Autodesk Inventor part; units mm, degrees
ref_plane "Work Plane1" through (55.8263, 1.3, -122.3626) normal (1, 0, 0) x (0, 0, -1)
ref_plane "Work Plane2" through (56.5713, 0, -122.3626) normal (-1, 0, 0) x (0, 0, 1)
ref_plane "Work Plane3" through (0, 0.5, 0) normal (0, -1, 0) x (1, 0, 0)
sketch "Sketch1" plane through (0, 0, 0) normal (0, 1, 0) x (-1, 0, 0)
  line L0 (-52.5263, -125.0626) -> (-59.1263, -125.0626)
  line L1 (-59.1263, -125.0626) -> (-59.1263, -122.3626)
  line L2 (-59.1263, -122.3626) -> (-52.5263, -122.3626)
  line L3 (-52.5263, -122.3626) -> (-52.5263, -125.0626)
  dimension "d0" = 6.6
  dimension "d1" = 2.7
extrude "Extrusion1" add sketch "Sketch1" along normal blind 1.3
sketch "Sketch2" plane through (52.5263, 0, -122.3626) normal (0, 0, 1) x (1, 0, 0)
  line L0 (6.6, 0) -> (6.6, 1.3)
  line L1 (6.6, 1.3) -> (4.67, 1.3)
  line L2 (0, 1.3) -> (6.6, 1.3)
  line L3 (0, 0) -> (6.6, 0)
  line L4 (4.67, 0) -> (3.42, 0)
  line L5 (3.42, 0) -> (3.42, 1)
  line L6 (3.42, 1) -> (4.67, 1)
  line L7 (4.67, 1) -> (4.67, 0)
  point P0 (3.42, 0)
  dimension "d4" = 1.93
  dimension "d5" = 1.25
  dimension "d6" = 1
extrude "Extrusion2" add sketch "Sketch2" along normal blind 1.5
sketch "Sketch3" plane through (0, 0, 0) normal (0, -1, 0) x (1, 0, 0)
  line L0 (55.8263, -125.0626) -> (55.8263, -126.2505)
  line L1 (52.5263, -125.0626) -> (52.0463, -125.0626)
  line L2 (52.0463, -125.0626) -> (52.0463, -124.6026)
  line L3 (52.0463, -124.6026) -> (52.5263, -124.6026)
  line L4 (52.5263, -122.3626) -> (52.0463, -122.3626)
  line L5 (52.0463, -122.3626) -> (52.0463, -122.8226)
  line L6 (52.0463, -122.8226) -> (52.5263, -122.8226)
  line L7 (59.1263, -125.0626) -> (59.6063, -125.0626)
  line L8 (59.6063, -125.0626) -> (59.6063, -124.6026)
  line L9 (59.6063, -124.6026) -> (59.1263, -124.6026)
  line L10 (59.1263, -122.3626) -> (59.6063, -122.3626)
  line L11 (59.6063, -122.3626) -> (59.6063, -122.8226)
  line L12 (59.6063, -122.8226) -> (59.1263, -122.8226)
  line L13 (52.5263, -126.3425) -> (53.2263, -126.3425)
  line L14 (59.1263, -125.0626) -> (59.1263, -125.9026)
  line L15 (59.1263, -122.3626) -> (59.1263, -122.8226)
  line L16 (59.1263, -124.6026) -> (59.1263, -125.0626)
  line L17 (52.5263, -125.0626) -> (52.5263, -124.6026)
  line L18 (52.5263, -122.8226) -> (52.5263, -122.3626)
  line L19 (59.1263, -125.0626) -> (52.5263, -125.0626)
  line L20 (53.2263, -125.9026) -> (53.6263, -125.9026)
  line L21 (53.6263, -125.9026) -> (53.6263, -125.0626)
  line L22 (53.6263, -125.0626) -> (53.2263, -125.0626)
  line L23 (53.2263, -125.0626) -> (53.2263, -125.9026)
  line L24 (58.4263, -125.9026) -> (58.0263, -125.9026)
  line L25 (58.0263, -125.9026) -> (58.0263, -125.0626)
  line L26 (58.0263, -125.0626) -> (58.4263, -125.0626)
  line L27 (58.4263, -125.0626) -> (58.4263, -125.9026)
  line L28 (58.0263, -125.9026) -> (57.0263, -125.9026)
  line L29 (56.6263, -125.0626) -> (57.0263, -125.0626)
  line L30 (57.0263, -125.0626) -> (57.0263, -125.9026)
  line L31 (56.6263, -125.9026) -> (56.6263, -125.0626)
  line L32 (57.0263, -125.9026) -> (56.6263, -125.9026)
  dimension "d15" = 0.4
  dimension "d16" = 1
extrude "Extrusion3" add sketch "Sketch3" against normal blind 0.2 contours L1 L2 L3 L17 | L16 L9 L8 L7 | L19 L30 L32 L31 | L19 L21 L20 L23 | L19 L27 L24 L25 | L18 L6 L5 L4 | L10 L11 L12 L15
ref_plane "Work Plane1" through (55.8263, 1.3, -122.3626) normal (1, 0, 0) x (0, 0, -1)
ref_plane "Work Plane2" through (56.5713, 0, -122.3626) normal (-1, 0, 0) x (0, 0, 1)
ref_plane "Work Plane3" through (0, 0.5, 0) normal (0, -1, 0) x (1, 0, 0)
properties part number "Power Swicth"
Input: part model. Units: mm. Frame: model coordinates. A direction names the side the tool comes from. Give positions to 0.01 mm unless a question says otherwise; leave off trailing zeros. Write each loop counter-clockwise with the first axis right and the second up, starting at its lowest first coordinate (ties: lowest second). Pieces come first, ordered by that corner, then holes.
Q1. Material intervals for probe 1 along X at (y, z) = (1.25, -124.2); probe 2 along Z at (x, y) = (56.5, 1.15); probe 3 along X at (y, z) = (0.5, -122.1), sorted ascending.
Q2. Set-up query: faces 1 (the face through (56, 0, -124)), 2 (the face through (55.946, 0.5, -121.6)), 3 (the face through (56, 1.3, -124)), 4 (the face through (57.196, 0.5, -121.6)), 5 (the face through (57, 1, -122)). Return all of +Z, -Z, +X, -X, +Y, -Y with unobstructed straight access to the full face (end or side cutting, diameter ignored); none if empty.
Q3. Section A-A, the plane y = 0.85. Output: boundary loops of the cut face in (x, z), plus the area to 3 significant figures.
Q4. Section B-B, the plane z = -122.6. Output: boundary loops of the cut face in (x, y), plus the area to 3 significant figures.
Q5. Section C-C, the plane x = 53.5. Output: boundary loops of the cut face in (y, z).
Q6. First-contact query: P1, Ø0.6, axis at y = 1, z = -124, coming from the -X side. Flat tip, straight axial feed; report the tip coordinate or a pass-through.
Q7. Section D-D, the plane y = 0.1. Output: boundary loops of the cut face in (x, z).
Filled in:
1. probe 1: x = 52.53 to 59.13
1. probe 2: z = -125.06 to -122.36
1. probe 3: x = 55.95 to 57.2
2. face 1: +Z, -Z, +X, -X, -Y
2. face 2: +Z, -X, +Y, -Y
2. face 3: +Z, -Z, +X, -X, +Y
2. face 4: +Z, +X, +Y, -Y
2. face 5: +Z, +X, -X, +Y
3. outline: (52.53, -125.06) - (59.13, -125.06) - (59.13, -122.36) - (57.2, -122.36) - (57.2, -120.86) - (55.95, -120.86) - (55.95, -122.36) - (52.53, -122.36) - close
3. area: 19.7 mm2
4. outline: (52.05, 0) - (59.61, 0) - (59.61, 0.2) - (59.13, 0.2) - (59.13, 1.3) - (52.53, 1.3) - (52.53, 0.2) - (52.05, 0.2) - close
4. area: 8.77 mm2
5. outline: (0, -125.9) - (0.2, -125.9) - (0.2, -125.06) - (1.3, -125.06) - (1.3, -122.36) - (0, -122.36) - close
6. P1: stops at x = 52.53
7. outline: (52.05, -125.06) - (53.23, -125.06) - (53.23, -125.9) - (53.63, -125.9) - (53.63, -125.06) - (56.63, -125.06) - (56.63, -125.9) - (57.03, -125.9) - (57.03, -125.06) - (58.03, -125.06) - (58.03, -125.9) - (58.43, -125.9) - (58.43, -125.06) - (59.61, -125.06) - (59.61, -124.6) - (59.13, -124.6) - (59.13, -122.82) - (59.61, -122.82) - (59.61, -122.36) - (57.2, -122.36) - (57.2, -120.86) - (55.95, -120.86) - (55.95, -122.36) - (52.05, -122.36) - (52.05, -122.82) - (52.53, -122.82) - (52.53, -124.6) - (52.05, -124.6) - close
